from build123d import *

# Parameters (mm, degrees)
F0_W     = 40
F0_H     = 40
F1_DEPTH = 10
F2_D     = 2.2
F2_DEPTH = 40
F3_R     = 2
F4_R     = 14
F5_DEPTH = 1
F6_W     = 33.6
F6_H     = 7.6
F7_DEPTH = 5
F8_R     = 1.6
F9_DEPTH = 1


with BuildPart() as f1:
    # F0 (on Top) → F1 (new body)
    with BuildSketch(Plane.XY):
        Rectangle(F0_W, F0_H)
    extrude(amount=F1_DEPTH)

    # F2
    with Locations(Plane(origin=(0, 0, 0), x_dir=(1, 0, 0), z_dir=(0, 0, -1))):
        with Locations((-18, -18), (-18, 18), (18, 18), (18, -18)):
            Hole(F2_D / 2, depth=F2_DEPTH)

    # F3
    f3_edges = [f1.edges().sort_by_distance(p)[0] for p in [
        (-20, -20, 5),
        (-20, 20, 5),
        (20, -20, 5),
        (20, 20, 5),
    ]]
    fillet(f3_edges, radius=F3_R)

    # F4 (on face) → F5 (join)
    with BuildSketch(Plane.XY.offset(10)):
        with Locations((0, -3)):
            Circle(F4_R)
    extrude(amount=F5_DEPTH)

    # F6 (on face) → F7 (cut)
    with BuildSketch(Plane(origin=(-20, 0, 0), x_dir=(0, -1, 0), z_dir=(-1, 0, 0))):
        with Locations((0, 5)):
            Rectangle(F6_W, F6_H)
    extrude(amount=-F7_DEPTH, mode=Mode.SUBTRACT)

    # F8 (on face) → F9 (cut)
    with BuildSketch(Plane.XZ.offset(20)):
        with Locations((0, 5)):
            Circle(F8_R)
    extrude(amount=-F9_DEPTH, mode=Mode.SUBTRACT)


solid = f1.part
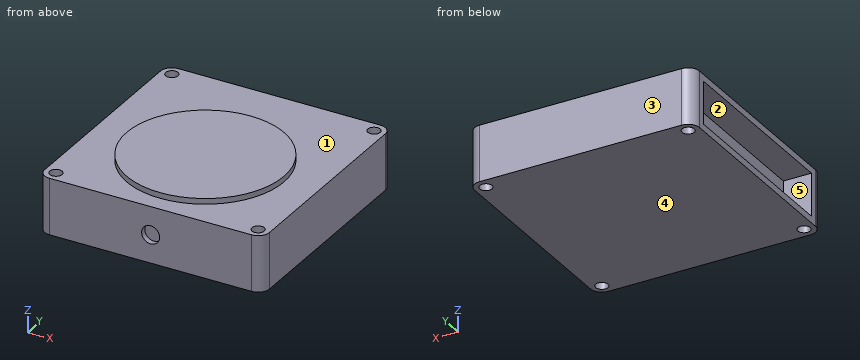
Read the model definition and answer for the solid it produces. Units are mm, in the model's axes. Face numbers are marked on the shaded views. A direction names the side the tool comes from. Coordinates: 2 decimals unless noted, no trailing zeros. Order: outer loops, then holes, each group sorted by start corner. A loop starts at its lowest first (then second) coordinate and runs counter-clockwise, first axis right, second up. Notation, with made-up numbers: M 70.25,53.25 L 104.25,53.25 A20 ccw 104.25,77.25 Z; hole C 73,34.5 d11. An arc over 180 degrees is marked long. Put each result on its own line as item: value. Start each with the question number.
Item 1: For the marked faces 4 and 5, determine the directions among +Z, -Z, +X, -X, +Y, -Y from which every point of the face is accessible in a straight line to the end or side of a thin tool.
Item 2: Given pin 1 Ø2.5 at (y, z) = (7.5, 3.5) entering from -X; pin 2 Ø1.6 at (x, z) = (-0.5, 5.5) entering from -Y; pin 3 Ø2 at (x, y) = (14.5, 10.5) entering from +Z; pin 4 Ø1.3 at (x, y) = (18, -18) entering from +Z, each flat-ended and moving along its own axis, determine where each tip first touches the part or whether it passes through.
Item 3: Section D-D, the plane z = 8.25 is taken. Determine the outline of the cut face in (x, y).
Item 4: Consider probe 1 along X at (y, z) = (-18, 7); probe 2 along Y at (x, z) = (-16, 6). Determine where each line is inside the solid, lowest interval first. Write a range as [from, to].
Item 5: The mould has two halves that part along Y. Classify the marked faces 1, 2 and 3: +Y half, -Y half, draft (parallel to the pull), parting line (faces both ways), or undercut.
Item 6: Section C-C, the plane x = 0 is taken. Determine the outline of the cut face in (y, z).
Item 7: Section B-B, the plane y = -3 is taken. Determine the outline of the cut face in (x, z), plus the area to 3 significant figures.
Item 8: Section A-A, the plane z = 5 is taken. Determine the outline of the cut face in (x, y), plus the area to 3 significant figures.
Computed:
1. face 4: -Z, +X, -X, +Y, -Y
1. face 5: -X
2. pin 1: stops at x = -15
2. pin 2: stops at y = -19
2. pin 3: stops at z = 10
2. pin 4: passes through
3. outline: M -20,-18 A2 ccw -18,-20 L 18,-20 A2 ccw 20,-18 L 20,18 A2 ccw 18,20 L -18,20 A2 ccw -20,18 L -20,16.8 L -15,16.8 L -15,-16.8 L -20,-16.8 Z; hole C -18,-18 d2.2; hole C -18,18 d2.2; hole C 18,-18 d2.2; hole C 18,18 d2.2
4. probe 1: x = [-20, -19.1], [-16.9, 16.9], [19.1, 20]
4. probe 2: y = [-20, -16.8], [16.8, 20]
5. face 1: draft
5. face 2: undercut
5. face 3: +Y half
6. outline: M -20,0 L 20,0 L 20,10 L 11,10 L 11,11 L -17,11 L -17,10 L -20,10 L -20,6.6 L -19,6.6 L -19,3.4 L -20,3.4 Z
7. outline: M -20,0 L 20,0 L 20,10 L 14,10 L 14,11 L -14,11 L -14,10 L -20,10 L -20,8.8 L -15,8.8 L -15,1.2 L -20,1.2 Z
7. area: 390 mm2
8. outline: M -20,-18 A2 ccw -18,-20 L -1.6,-20 L -1.6,-19 L 1.6,-19 L 1.6,-20 L 18,-20 A2 ccw 20,-18 L 20,18 A2 ccw 18,20 L -18,20 A2 ccw -20,18 L -20,16.8 L -15,16.8 L -15,-16.8 L -20,-16.8 Z; hole C -18,-18 d2.2; hole C -18,18 d2.2; hole C 18,-18 d2.2; hole C 18,18 d2.2
8. area: 1,410 mm2
